Build history of the part. All positions in model axes, mm. Give positions to 0.01 mm unless a question says otherwise; leave off trailing zeros. Write each loop counter-clockwise with the first axis right and the second up, starting at its lowest first coordinate (ties: lowest second). Pieces come first, ordered by that corner, then holes. Notation, with made-up numbers: (48.5, -9) -> (83.5, -9) arc R9 cw to (83.5, -5) -> close; hole circle Ø6 at (-0.75, 75). An arc over 180 degrees is marked (long way). Put each result on its own line as item: value.
Autodesk Inventor part; units mm, degrees
ref_plane "YZ Plane" through (0, 0, 0) normal (1, 0, 0) x (0, 1, 0)
ref_plane "XZ Plane" through (0, 0, 0) normal (0, 1, 0) x (-1, 0, 0)
ref_plane "XY Plane" through (0, 0, 0) normal (0, 0, 1) x (1, 0, 0)
sketch "Sketch1" plane through (0, 0, 0) normal (0, 0, 1) x (1, 0, 0)
  circle A0 centre (5.0002, 0) radius 1.25 construction
  line L0 (1.4779, -3) -> (1.4779, 3) construction
  line L1 (5.0002, -3) -> (1.4779, -3) construction
  arc A1 (5.0002, -3) -> (5.0002, 3) centre (5.0002, 0) ccw construction
  line L2 (1.4779, 3) -> (5.0002, 3) construction
  circle A2 centre (-5.0002, 0) radius 1.25 construction
  line L3 (-1.4614, 3) -> (-1.4614, -3) construction
  line L4 (-5.0002, 3) -> (-1.4614, 3) construction
  arc A3 (-5.0002, 3) -> (-5.0002, -3) centre (-5.0002, 0) ccw construction
  line L5 (-1.4614, -3) -> (-5.0002, -3) construction
  line L6 (-5.0002, 0) -> (5.0002, 0) construction
  line L7 (-5.0002, -2.75) -> (5.0002, -2.75)
  line L8 (5.0002, 2.75) -> (-5.0002, 2.75)
  arc A4 (-5.0002, 2.75) -> (-5.0002, -2.75) centre (-5.0002, 0) ccw
  arc A5 (5.0002, -2.75) -> (5.0002, 2.75) centre (5.0002, 0) ccw
  circle A6 centre (-5.0002, 0) radius 1.65
  circle A7 centre (5.0002, 0) radius 1.65
  point P0 (0, 0)
  point P1 (0, 0)
  dimension "d0" = 5.5
  dimension "d1" = 3.3
  dimension "d2" = 3.3
extrude "Extrusion1" add sketch "Sketch1" along normal blind 1.5
sketch "Sketch2" plane through (-5.0002, 2.75, 0) normal (0, 1, 0) x (1, 0, 0)
  circle A0 centre (5.0085, 1.8) radius 2.1
  arc A1 (5.0085, 3.6) -> (5.0085, -0.6) centre (5.0085, 1.5) ccw
  point P0 (5.0002, 0)
extrude "Extrusion2" cut sketch "Sketch2" against normal through all
properties part number "TubeClamp"
1) Slice it at B-B (x = 6). Write the cut outline in (y, z), plus the area to 3 significant figures.
Filled sheet:
outline: (-2.56, 0) -> (-1.31, 0) -> (-1.31, 1.5) -> (-2.56, 1.5) -> close; (1.31, 0) -> (2.56, 0) -> (2.56, 1.5) -> (1.31, 1.5) -> close
area: 3.75 mm2
2) Wall check: L1, parallel to X at y = -0.8, z = 0.55; L2, parallel to X at y = 1.05, z = 0.8; L3, parallel to Y at x = 6.5, z = 0.35. Give the ranges that are in metal, low to high.
Filled sheet:
L1: -7.63 to -6.44, -3.56 to 3.56, 6.44 to 7.63
L2: -7.54 to -6.27, -3.73 to 3.73, 6.27 to 7.54
L3: -2.31 to -0.69, 0.69 to 2.31
3) Pull direction X, two halves, no side cores. Call faces 1 (the cylindrical face through (3.35, -0.07, 0.74)), 2 (the cylindrical face through (7.75, 0.06, 0.74)), 3 (the cylindrical face through (-7.75, -0.06, 0.74)), 4 (the flat face through (3, 0, 0)): released by +X, released by -X, zero draft, split by the parting line, or undercut.
Filled sheet:
face 1: undercut
face 2: released by +X
face 3: released by -X
face 4: zero draft
4) Slice it at A-A (y = 0). Write the cut outline in (x, z).
Filled sheet:
outline: (-7.75, 0) -> (-6.65, 0) -> (-6.65, 1.5) -> (-7.75, 1.5) -> close; (-3.35, 0) -> (-1.07, 0) arc R2.1 cw to (1.09, 0) -> (3.35, 0) -> (3.35, 1.5) -> (-3.35, 1.5) -> close; (6.65, 0) -> (7.75, 0) -> (7.75, 1.5) -> (6.65, 1.5) -> close
5) Slice it at C-C (z = 1.05). Write the cut outline in (x, y), plus the area to 3 significant figures.
Filled sheet:
outline: (-5, -2.75) -> (5, -2.75) arc R2.75 ccw to (5, 2.75) -> (-5, 2.75) arc R2.75 ccw to start; hole circle Ø3.3 at (-5, 0); hole circle Ø3.3 at (5, 0)
area: 61.7 mm2
6) Slice it at D-D (y = 0.8). Write the cut outline in (x, z).
Filled sheet:
outline: (-7.63, 0) -> (-6.44, 0) -> (-6.44, 1.5) -> (-7.63, 1.5) -> close; (-3.56, 0) -> (-1.07, 0) arc R2.1 cw to (1.09, 0) -> (3.56, 0) -> (3.56, 1.5) -> (-3.56, 1.5) -> close; (6.44, 0) -> (7.63, 0) -> (7.63, 1.5) -> (6.44, 1.5) -> close
